Source: CAD feature listing. Evaluate the final solid. Frame: model axes, mm. Round coordinates to 2 decimals unless told otherwise and drop trailing zeros. Write each loop counter-clockwise with the first axis right and the second up, starting at its lowest first coordinate (ties: lowest second). Pieces come first, ordered by that corner, then holes. Notation, with made-up numbers: M 48,22 L 69,22 A30 cw 69,56 Z; hole C 62.5,30.25 d8. An arc over 180 degrees is marked long. Use a Markdown table: item, result.
```python
from build123d import *
from OCP.BRepFilletAPI import BRepFilletAPI_MakeChamfer

# Parameters (mm, degrees)
BOSS_EXTRUDE1_DEPTH = 3
SKETCH2_R           = 1.5
CUT_EXTRUDE1_DEPTH  = 103.574363269
CHAMFER1_SIZE       = 1.5
CHAMFER1_SIZE2      = 1.303930107
CUT_EXTRUDE2_DEPTH  = 103.574363269
SKETCH4_W           = 20
SKETCH4_H           = 1.7
CUT_EXTRUDE3_DEPTH  = 103.574363269
SKETCH5_R           = 5
CUT_EXTRUDE4_DEPTH  = 103.085748271


with BuildPart() as part:
    # Sketch1 → Boss-Extrude1 (new body)
    with BuildSketch(Plane(origin=(0, 0, 0), x_dir=(1, 0, 0), z_dir=(0, 1, 0))):
        with BuildLine():
            Line((30.029977361, -64.812867647), (-30.029977361, -64.812867647))
            ThreePointArc((-30.029977361, -64.812867647), (-32.509837414, -64.500503794), (-34.834773739, -63.582926471))
            ThreePointArc((-34.834773739, -63.582926471), (0, 72.5), (34.834773739, -63.582926471))
            ThreePointArc((34.834773739, -63.582926471), (32.509837414, -64.500503794), (30.029977361, -64.812867647))
        make_face()
    extrude(amount=BOSS_EXTRUDE1_DEPTH)

    # Sketch2 → Cut-Extrude1 (cut, through all)
    with BuildSketch(Plane(origin=(0, 3, 0), x_dir=(1, 0, 0), z_dir=(0, 1, 0))):
        with Locations(Location((-30.5, 44, 0), (0, 0, 270))):
            Circle(SKETCH2_R)
        with Locations(Location((30.5, 44, 0), (0, 0, 270))):
            Circle(SKETCH2_R)
        with Locations(Location((30.5, 0, 0), (0, 0, 270))):
            Circle(SKETCH2_R)
        with Locations(Location((30.5, -44, 0), (0, 0, 270))):
            Circle(SKETCH2_R)
        with Locations(Location((-30.5, -44, 0), (0, 0, 270))):
            Circle(SKETCH2_R)
        with Locations(Location((-30.5, 0, 0), (0, 0, 270))):
            Circle(SKETCH2_R)
    extrude(amount=-CUT_EXTRUDE1_DEPTH, mode=Mode.SUBTRACT)

    # Chamfer1: one chamfer whose edges measure the first distance from different faces: ONE call of the kernel's chamfer builder (chamfer() names one face for all edges)
    chamfer1_edges_1 = [part.edges().sort_by_distance(p)[0] for p in [
        (-30.5, 3, -45.5),
    ]]
    chamfer1_side_1 = [part.faces().sort_by_distance(p)[0] for p in [
        (-30.5, 1.5, -45.5),
    ]]
    chamfer1_edges_2 = [part.edges().sort_by_distance(p)[0] for p in [
        (-30.5, 3, -1.5),
    ]]
    chamfer1_side_2 = [part.faces().sort_by_distance(p)[0] for p in [
        (-30.5, 1.5, -1.5),
    ]]
    chamfer1_edges_3 = [part.edges().sort_by_distance(p)[0] for p in [
        (-30.5, 3, 42.5),
    ]]
    chamfer1_side_3 = [part.faces().sort_by_distance(p)[0] for p in [
        (-30.5, 1.5, 42.5),
    ]]
    chamfer1_edges_4 = [part.edges().sort_by_distance(p)[0] for p in [
        (30.5, 3, 42.5),
    ]]
    chamfer1_side_4 = [part.faces().sort_by_distance(p)[0] for p in [
        (30.5, 1.5, 42.5),
    ]]
    chamfer1_edges_5 = [part.edges().sort_by_distance(p)[0] for p in [
        (30.5, 3, -1.5),
    ]]
    chamfer1_side_5 = [part.faces().sort_by_distance(p)[0] for p in [
        (30.5, 1.5, -1.5),
    ]]
    chamfer1_edges_6 = [part.edges().sort_by_distance(p)[0] for p in [
        (30.5, 3, -45.5),
    ]]
    chamfer1_side_6 = [part.faces().sort_by_distance(p)[0] for p in [
        (30.5, 1.5, -45.5),
    ]]
    chamfer1 = BRepFilletAPI_MakeChamfer(part.part.solid().wrapped)
    for e in chamfer1_edges_1:
        chamfer1.Add(CHAMFER1_SIZE, CHAMFER1_SIZE2, e.wrapped, chamfer1_side_1[0].wrapped)  # the first distance lies on this face
    for e in chamfer1_edges_2:
        chamfer1.Add(CHAMFER1_SIZE, CHAMFER1_SIZE2, e.wrapped, chamfer1_side_2[0].wrapped)  # the first distance lies on this face
    for e in chamfer1_edges_3:
        chamfer1.Add(CHAMFER1_SIZE, CHAMFER1_SIZE2, e.wrapped, chamfer1_side_3[0].wrapped)  # the first distance lies on this face
    for e in chamfer1_edges_4:
        chamfer1.Add(CHAMFER1_SIZE, CHAMFER1_SIZE2, e.wrapped, chamfer1_side_4[0].wrapped)  # the first distance lies on this face
    for e in chamfer1_edges_5:
        chamfer1.Add(CHAMFER1_SIZE, CHAMFER1_SIZE2, e.wrapped, chamfer1_side_5[0].wrapped)  # the first distance lies on this face
    for e in chamfer1_edges_6:
        chamfer1.Add(CHAMFER1_SIZE, CHAMFER1_SIZE2, e.wrapped, chamfer1_side_6[0].wrapped)  # the first distance lies on this face
    add(Compound.cast(chamfer1.Shape()), mode=Mode.REPLACE)

    # Sketch3 → Cut-Extrude2 (cut, through all)
    with BuildSketch(Plane(origin=(0, 3, 0), x_dir=(1, 0, 0), z_dir=(0, 1, 0))):
        Polygon((1.35, -61.812867647), (3.1, -61.812867647), (3.1, -59.612867647), (1.35, -59.612867647), (1.35, -55.812867647), (-1.35, -55.812867647), (-1.35, -59.612867647), (-3.1, -59.612867647), (-3.1, -61.812867647), (-1.35, -61.812867647), (-1.35, -64.812867647), (1.35, -64.812867647), align=None)
    extrude(amount=-CUT_EXTRUDE2_DEPTH, mode=Mode.SUBTRACT)

    # Sketch4 → Cut-Extrude3 (cut, through all)
    with BuildSketch(Plane(origin=(0, 3, 0), x_dir=(1, 0, 0), z_dir=(0, 1, 0))):
        with Locations((0, 70.957033082)):
            Rectangle(SKETCH4_W, SKETCH4_H)
    extrude(amount=-CUT_EXTRUDE3_DEPTH, mode=Mode.SUBTRACT)


with BuildPart() as body_2:
    # of the pieces the cut leaves, the one that is kept (cut_extrude3_keep)
    add(part.part.solids().sort_by_distance((-30.029977361, 3, 64.812867647))[0])

    # Sketch5 → Cut-Extrude4 (cut, through all)
    with BuildSketch(Plane(origin=(0, 3, 0), x_dir=(1, 0, 0), z_dir=(0, 1, 0))):
        with Locations(Location((0, 65, 0), (0, 0, 270))):
            Circle(SKETCH5_R)
        with Locations(Location((30, -57, 0), (0, 0, 90))):
            Circle(SKETCH5_R)
        with Locations(Location((-30, -57, 0), (0, 0, 270))):
            Circle(SKETCH5_R)
    extrude(amount=-CUT_EXTRUDE4_DEPTH, mode=Mode.SUBTRACT)


solid = body_2.part
```
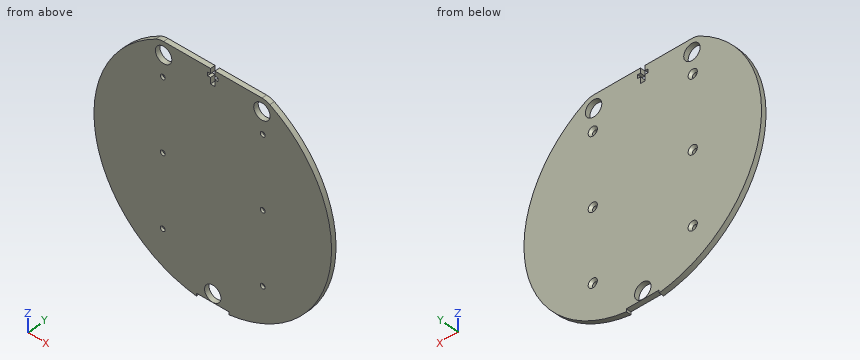
Q1. Section B-B on z = 35. Return loops of the section in (x, y), plus the area to 3 significant figures.
Results are:
| item | result |
|---|---|
| outline | M -63.49,0 L 63.49,0 L 63.49,3 L -63.49,3 Z |
| area | 381 mm^2 |
Q2. Section A-A on y = 1.05. Give the number of separate pieces and of enclosed holes in the cut face, plus the area to 3 significant figures.
Results are:
| item | result |
|---|---|
| separate pieces | 1 |
| enclosed holes | 9 |
| area | 15,800 mm^2 |
Q3. Line query: L1, parallel to X at y = 1.25, z = 44; L2, parallel to X at y = 0.4, z = 55; L3, parallel to X at y = 1.9, z = 57. Output: solid intervals per line, ascending.
Results are:
| item | result |
|---|---|
| L1 | -57.62 to -32, -29 to 29, 32 to 57.62 |
| L2 | -47.24 to -34.58, -25.42 to 25.42, 34.58 to 47.24 |
| L3 | -44.8 to -35, -25 to -1.35, 1.35 to 25, 35 to 44.8 |
Q4. First-contact query: pin 1 Ø4 at (x, z) = (30.5, -44) entering from +Y; pin 2 Ø3.5 at (x, z) = (-30.5, 0) entering from +Y; pin 3 Ø0.8 at (x, y) = (0.5, 1.5) entering from +Z. Flat tips, straight axial feed; report the tip coordinate or a pass-through.
Results are:
| item | result |
|---|---|
| pin 1 | y = 2.08 |
| pin 2 | y = 1.79 |
| pin 3 | z = 55.81 |
Q5. Section C-C on z = 49. Return loops of the section in (x, y).
Results are:
| item | result |
|---|---|
| outline | M -53.43,0 L 53.43,0 L 53.43,3 L -53.43,3 Z |
